```python
from build123d import *

# Parameters (mm, degrees)
F0_R     = 137.2744361776
F1_DEPTH = 177.8
F2_T     = 25.4


# Not quite as in the source:
# - a fillet or chamfer that OpenCascade refuses, or shapes differently, is made with other operations: its cross-section is extruded or revolved along the edge and cut away or added


with BuildPart() as f1:
    # F0 (on Front) → F1 (new body)
    with BuildSketch(Plane.XZ):
        with Locations((-6.2283538282, -7.7867358923)):
            Circle(F0_R)
    extrude(amount=F1_DEPTH)

    # F2
    f2_openings = [f1.faces().sort_by_distance(p)[0] for p in [
        (-6.228354, -177.8, -7.786736),
        (-6.228354, 0, -7.786736),
    ]]
    offset(amount=F2_T, openings=f2_openings)

    # F3: fillet of radius 25.4 on 2 edges, made by hand

    # F3_s1 → F3_t2 (revolve, cut)
    with BuildSketch(Plane.XY.offset(-7.7867358923)):
        with BuildLine():
            ThreePointArc((131.0460823494, 0), (149.0065945915, -7.4394877579), (156.4460823494, -25.4))
            Line((156.4460823494, -25.4), (156.4460823494, 0))
            Line((156.4460823494, 0), (131.0460823494, 0))
        make_face()
    revolve(axis=Axis((-6.2283538282, 0, -7.7867358923), (0, -1, 0)), mode=Mode.SUBTRACT)

    # F3_s3 → F3_t4 (revolve, cut)
    with BuildSketch(Plane.XY.offset(-7.7867358923)):
        with BuildLine():
            ThreePointArc((156.4460823494, -152.4), (149.0065945915, -170.3605122421), (131.0460823494, -177.8))
            Line((131.0460823494, -177.8), (156.4460823494, -177.8))
            Line((156.4460823494, -177.8), (156.4460823494, -152.4))
        make_face()
    revolve(axis=Axis((-6.2283538282, -177.8, -7.7867358923), (0, -1, 0)), mode=Mode.SUBTRACT)


solid = f1.part
```
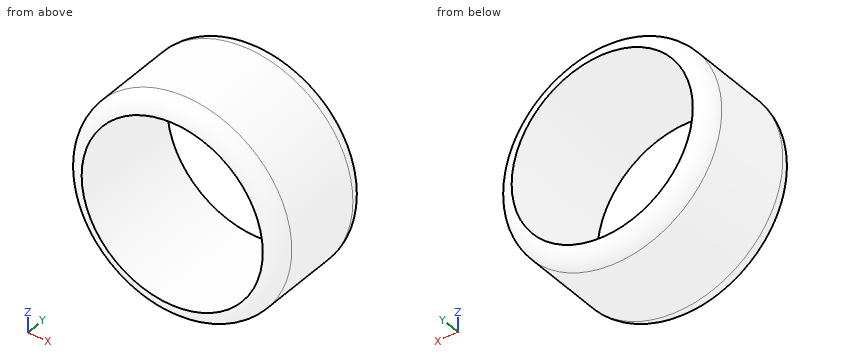
Geometry: final body of the model. Coordinates: model frame, mm. Coordinates: 2 decimals unless noted, no trailing zeros. Order: outer loops, then holes, each group sorted by start corner. A loop starts at its lowest first (then second) coordinate and runs counter-clockwise, first axis right, second up. Notation, with made-up numbers: (-2, 7) -> (33, 7) arc R13 cw to (33, 14) -> close; hole circle Ø3 at (88.5, 43.25). An arc over 180 degrees is marked (long way). Write each question's results on one line, items separated by ' | '. Start each with the question number.
1) Cut plane A-A, the plane y = -119. Output: boundary loops of the cut face in (x, z), and give its area (3 significant figures).
2) Material intervals for line 1 along Z through (x, y) = (-131.5, -116); line 2 along X through (y, z) = (-98.5, 72.5); line 3 along X through (y, z) = (-65.5, -4), sorted ascending.
3) First-contact query: pin 1 (10 mm diameter, centred on x = -57, y = -60, fed in from +Z); pin 2 (1.5 mm diameter, centred on x = -119, y = -19.5, fed in from +Z); pin 3 (1 mm diameter, centred on y = -108.5, z = -82.5, fed in from -X). Flat tips, straight axial feed; report the tip coordinate or a pass-through.
Checks:
1) outline: circle Ø325.35 at (-6.23, -7.79); hole circle Ø274.55 at (-6.23, -7.79) | area: 23,900 mm^2
2) line 1: -111.57 to -63.92, 48.35 to 95.99 | line 2: -147.71 to -117.58, 105.12 to 135.25 | line 3: -168.86 to -143.45, 130.99 to 156.4
3) pin 1: z = 148.32 | pin 2: z = 109.25 | pin 3: x = -150.99
